Read the model definition and answer for the solid it produces. Units are mm, in the model's axes. A direction names the side the tool comes from. Round coordinates to 2 decimals unless told otherwise and drop trailing zeros. Loops run counter-clockwise (first coordinate to the right, second up) from the corner with the lowest first, then second, coordinate; pieces in that order, holes last. Notation, with made-up numbers: M 60,12.5 L 76,12.5 A13 cw 76,23.5 Z; hole C 9.5,78 d2. An arc over 180 degrees is marked long. Write each question's results on one line, items separated by ' | '.
from build123d import *

# Parameters (mm, degrees)
SKETCH1_W           = 40
SKETCH1_H           = 40
BOSS_EXTRUDE1_DEPTH = 10
SKETCH2_R           = 2.2
CUT_EXTRUDE1_DEPTH  = 10
SKETCH3_R           = 19.2
CUT_EXTRUDE2_DEPTH  = 10
FILLET1_R           = 4.4
BOSS_EXTRUDE2_DEPTH = 1.5


with BuildPart() as part:
    # Sketch1 → Boss-Extrude1 (new body)
    with BuildSketch(Plane.XY):
        Rectangle(SKETCH1_W, SKETCH1_H)
    extrude(amount=BOSS_EXTRUDE1_DEPTH)

    # Sketch2 → Cut-Extrude1 (cut)
    with BuildSketch(Plane.XY.offset(10)):
        with Locations((-16, 16)):
            Circle(SKETCH2_R)
        with Locations((16, 16)):
            Circle(SKETCH2_R)
        with Locations((16, -16)):
            Circle(SKETCH2_R)
        with Locations((-16, -16)):
            Circle(SKETCH2_R)
    extrude(amount=-CUT_EXTRUDE1_DEPTH, mode=Mode.SUBTRACT)

    # Sketch3 → Cut-Extrude2 (cut)
    with BuildSketch(Plane.XY.offset(10)):
        Circle(SKETCH3_R)
    extrude(amount=-CUT_EXTRUDE2_DEPTH, mode=Mode.SUBTRACT)

    # Fillet1
    fillet1_edges = [part.edges().sort_by_distance(p)[0] for p in [
        (-20, 20, 5),
        (20, 20, 5),
        (20, -20, 5),
        (-20, -20, 5),
    ]]
    fillet(fillet1_edges, radius=FILLET1_R)

    # Sketch4 → Boss-Extrude2 (add)
    with BuildSketch(Plane.XY.offset(10)):
        with BuildLine():
            Line((6.50980229, 8.866931496), (-6.175215064, 18.179843754))
            ThreePointArc((-6.175215064, 18.179843754), (-7.1684264, 17.811615956), (-8.139818596, 17.389173449))
            Line((-8.139818596, 17.389173449), (0.583931442, 10.98449016))
            ThreePointArc((0.583931442, 10.98449016), (-4.707199842, 9.941944963), (-8.866931496, 6.50980229))
            Line((-8.866931496, 6.50980229), (-18.179843754, -6.175215064))
            ThreePointArc((-18.179843754, -6.175215064), (-17.811615956, -7.1684264), (-17.389173449, -8.139818596))
            Line((-17.389173449, -8.139818596), (-10.98449016, 0.583931442))
            ThreePointArc((-10.98449016, 0.583931442), (-9.941944963, -4.707199842), (-6.50980229, -8.866931496))
            Line((-6.50980229, -8.866931496), (6.175215064, -18.179843754))
            ThreePointArc((6.175215064, -18.179843754), (7.1684264, -17.811615956), (8.139818596, -17.389173449))
            Line((8.139818596, -17.389173449), (-0.583931442, -10.98449016))
            ThreePointArc((-0.583931442, -10.98449016), (4.707199842, -9.941944963), (8.866931496, -6.50980229))
            Line((8.866931496, -6.50980229), (18.179843754, 6.175215064))
            ThreePointArc((18.179843754, 6.175215064), (17.811615956, 7.1684264), (17.389173449, 8.139818596))
            Line((17.389173449, 8.139818596), (10.98449016, -0.583931442))
            ThreePointArc((10.98449016, -0.583931442), (9.941944963, 4.707199842), (6.50980229, 8.866931496))
        make_face()
    extrude(amount=-BOSS_EXTRUDE2_DEPTH)


solid = part.part
Item 1: The mould has two halves that part along X. Classify faces 3 (the face through (18.677, -18.745, 5.07)), 4 (the face through (-13.968, -16.843, 5.07)), 5 (the face through (-8, 18, 0)): pulls with the +X half, pulls with the -X half, needs draft (parallel to the pull), parting line crosses it, or undercut.
Outcome:
face 3: pulls with the +X half | face 4: undercut | face 5: needs draft
Item 2: The part is cut by section A-A (z = 6). Determine the outline of the cut face in (x, y).
Outcome:
outline: M -20,-15.6 A4.4 ccw -15.6,-20 L 15.6,-20 A4.4 ccw 20,-15.6 L 20,15.6 A4.4 ccw 15.6,20 L -15.6,20 A4.4 ccw -20,15.6 Z; hole C 0,0 d38.4; hole C -16,-16 d4.4; hole C -16,16 d4.4; hole C 16,-16 d4.4; hole C 16,16 d4.4
Item 3: The part is cut by section D-D (y = -14.5). Determine the outline of the cut face in (x, z), plus the area to 3 significant figures.
Outcome:
outline: M -20,0 L -17.61,0 L -17.61,10 L -20,10 Z; M -14.39,0 L -12.59,0 L -12.59,10 L -14.39,10 Z; M 1.16,8.5 L 4.2,8.5 L 4.2,10 L 1.16,10 Z; M 12.59,0 L 14.39,0 L 14.39,10 L 12.59,10 Z; M 17.61,0 L 20,0 L 20,10 L 17.61,10 Z | area: 88.5 mm2
Item 4: Flat-ended cylindrical pins translate along their axes: pin 1 (3.5 mm diameter, centred on x = 16, y = 16, fed in from +Z); pin 2 (6 mm diameter, centred on x = 9.5, y = -8.5, fed in from -Z). Find the tip coordinate at first contact, or state that the pin passes through.
Outcome:
pin 1: passes through | pin 2: stops at z = 8.5
Item 5: For faces 1 (the face through (0, 0, 10)), 2 (the face through (13.458, -0.256, 9.26)), determine the directions among +Z, -Z, +X, -X, +Y, -Y from which every point of the face is accessible in a straight line to the end or side of a thin tool.
Outcome:
face 1: +Z, +X, -X, +Y, -Y | face 2: +Z, -Z
Item 6: The part is cut by section C-C (y = 10). Determine the outline of the cut face in (x, z).
Outcome:
outline: M -20,0 L -16.39,0 L -16.39,10 L -20,10 Z; M -4.58,8.5 L 4.97,8.5 L 4.97,10 L -4.58,10 Z; M 16.39,0 L 20,0 L 20,10 L 16.39,10 Z
Item 7: The part is cut by section B-B (x = 2). Determine the outline of the cut face in (y, z).
Outcome:
outline: M -20,0 L -19.1,0 L -19.1,10 L -20,10 Z; M -15.11,8.5 L -12.88,8.5 L -12.88,10 L -15.11,10 Z; M -10.82,8.5 L 12.18,8.5 L 12.18,10 L -10.82,10 Z; M 19.1,0 L 20,0 L 20,10 L 19.1,10 Z
Item 8: Straight lines are drawn through the part: line 1 (Y direction, x = -16, z = 7.5); line 2 (X direction, y = -13, z = 9.25); line 3 (X direction, y = 15.5, z = 1.5). For each, find the intervals that lie inside material, in ascending order.
Outcome:
line 1: y = -19.98 to -18.2, -13.8 to -10.61, 10.61 to 13.8, 18.2 to 19.98 | line 2: x = -20 to -14.13, -0.88 to 2.16, 14.13 to 20 | line 3: x = -20 to -18.14, -13.86 to -11.33, 11.33 to 13.86, 18.14 to 20
